Source: CAD feature listing. Evaluate the final solid. Frame: model axes, mm. Round coordinates to 2 decimals unless told otherwise and drop trailing zeros. Write each loop counter-clockwise with the first axis right and the second up, starting at its lowest first coordinate (ties: lowest second). Pieces come first, ordered by that corner, then holes. Notation, with made-up numbers: M -33,74 L -28,74 A23 ccw -28,95 Z; hole C -37.75,45.5 d3. An arc over 180 degrees is marked long. Use a Markdown table: item, result.
```python
from build123d import *

# Parameters (mm, degrees)
SKETCH2_R           = 2.5
SKETCH2_R_2         = 19
SKETCH2_R_3         = 5
SKETCH2_R_4         = 2
BOSS_EXTRUDE2_DEPTH = 6


with BuildPart() as part:
    # Sketch2 → Boss-Extrude2 (new body)
    with BuildSketch(Plane.XY):
        with BuildLine():
            Line((-69.048275573, 22), (70, 22))
            Line((70, 22), (70, 47.4))
            Line((70, 47.4), (83.667882182, 56.970354135))
            ThreePointArc((83.667882182, 56.970354135), (85.235054166, 58.75737129), (85.8, 61.066114356))
            Line((85.8, 61.066114356), (85.8, 100))
            ThreePointArc((85.8, 100), (84.335533906, 103.535533906), (80.8, 105))
            Line((80.8, 105), (-18.818802154, 105))
            Line((-18.818802154, 105), (-49.04048999, 157.345498823))
            ThreePointArc((-49.04048999, 157.345498823), (-52.700744028, 161.005752861), (-57.700744028, 162.345498823))
            Line((-57.700744028, 162.345498823), (-95.228511525, 162.345498823))
            ThreePointArc((-95.228511525, 162.345498823), (-100.228511525, 161.005752861), (-103.888765563, 157.345498823))
            Line((-103.888765563, 157.345498823), (-122.652649312, 124.845498823))
            ThreePointArc((-122.652649312, 124.845498823), (-123.992395274, 119.845498823), (-122.652649312, 114.845498823))
            Line((-122.652649312, 114.845498823), (-69.048275573, 22))
        make_face()
        with Locations((-11.557721787, 45.22)):
            Circle(SKETCH2_R, mode=Mode.SUBTRACT)
        with Locations((35.582278213, 45.22)):
            Circle(SKETCH2_R, mode=Mode.SUBTRACT)
        with Locations((35.582278213, 92.36)):
            Circle(SKETCH2_R, mode=Mode.SUBTRACT)
        with Locations((12.012278213, 68.79)):
            Circle(SKETCH2_R_2, mode=Mode.SUBTRACT)
        with Locations((-11.557721787, 92.36)):
            Circle(SKETCH2_R, mode=Mode.SUBTRACT)
        with Locations((-46.987721787, 68.79)):
            Circle(SKETCH2_R_3, mode=Mode.SUBTRACT)
        with Locations((-38.936860279, 119.845498823)):
            Circle(SKETCH2_R_4, mode=Mode.SUBTRACT)
        with Locations((-95.228511525, 87.345498823)):
            Circle(SKETCH2_R_4, mode=Mode.SUBTRACT)
        with Locations((-76.464627777, 119.845498823)):
            Circle(SKETCH2_R_3, mode=Mode.SUBTRACT)
        with Locations((-95.228511525, 152.345498823)):
            Circle(SKETCH2_R_4, mode=Mode.SUBTRACT)
    extrude(amount=BOSS_EXTRUDE2_DEPTH)


solid = part.part
```
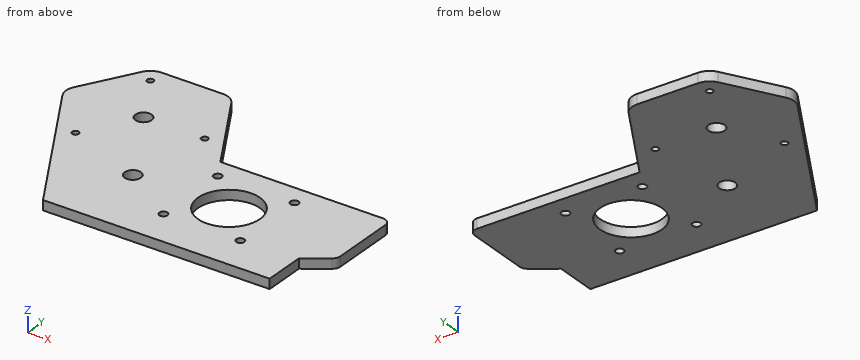
Q1. Section B-B on x = 25.5. Return loops of the section in (y, z), plus the area to 3 significant figures.
Results are:
| item | result |
|---|---|
| outline | M 22,0 L 55.41,0 L 55.41,6 L 22,6 Z; M 82.17,0 L 105,0 L 105,6 L 82.17,6 Z |
| area | 337 mm^2 |
Q2. Section A-A on y = 68.79. Return loops of the section in (x, z).
Results are:
| item | result |
|---|---|
| outline | M -96.06,0 L -51.99,0 L -51.99,6 L -96.06,6 Z; M -41.99,0 L -6.99,0 L -6.99,6 L -41.99,6 Z; M 31.01,0 L 85.8,0 L 85.8,6 L 31.01,6 Z |
Q3. Line query: L1, parallel to Y at x = -94.5, z = 3.85; L2, parallel to Y at x = -17, z = 2.85; L3, parallel to X at y = 61, z = 2.6. Output: solid intervals per line, ascending.
Results are:
| item | result |
|---|---|
| L1 | 66.08 to 85.48, 89.21 to 150.48, 154.21 to 162.35 |
| L2 | 22 to 105 |
| L3 | -91.56 to -5.32, 29.34 to 85.8 |
Q4. Section D-D on y = 92.36. Return loops of the section in (x, z), plus the area to 3 significant figures.
Results are:
| item | result |
|---|---|
| outline | M -109.67,0 L -14.06,0 L -14.06,6 L -109.67,6 Z; M -9.06,0 L 33.08,0 L 33.08,6 L -9.06,6 Z; M 38.08,0 L 85.8,0 L 85.8,6 L 38.08,6 Z |
| area | 1,110 mm^2 |
Q5. Section C-C on z = 2.25. Give the number of separate pieces and of enclosed holes in the cut face, plus the area to 3 significant figures.
Results are:
| item | result |
|---|---|
| separate pieces | 1 |
| enclosed holes | 10 |
| area | 17,500 mm^2 |
Q6. First-contact query: pin 1 Ø8 at (x, y) = (-76.46, 119.85) entering from +Z; pin 2 Ø3 at (y, z) = (41, 1.5) entering from +X. Flat tips, straight axial feed; report the tip coordinate or a pass-through.
Results are:
| item | result |
|---|---|
| pin 1 | through |
| pin 2 | x = 70 |
